For this review, take the finished solid that the model builds, in its own axes (mm). Round coordinates to 2 decimals unless told otherwise and drop trailing zeros. Write each loop counter-clockwise with the first axis right and the second up, starting at its lowest first coordinate (ties: lowest second). Pieces come first, ordered by that corner, then holes. Notation, with made-up numbers: (33.5, -38.75) -> (40.5, -38.75) arc R18 cw to (40.5, -15.75) -> close; hole circle Ø3 at (45.25, 81.5). An arc over 180 degrees is marked (long way). Answer in a Markdown table with one row per item. Add a question column.
```python
from build123d import *

# Parameters (mm, degrees)
SZKIC1_R                    = 1.5
SZKIC1_W                    = 45
SZKIC1_H                    = 5
SZKIC1_W_2                  = 5
SZKIC1_H_2                  = 55
DODANIE_WYCI_GNI_CIE3_DEPTH = 2


with BuildPart() as part:
    # Szkic1 → Dodanie-wyciągnięcie3 (new body)
    with BuildSketch(Plane.XY):
        with BuildLine():
            Line((-139.727293062, -79.5), (-120.189002398, -79.5))
            ThreePointArc((-120.189002398, -79.5), (-117.912369122, -78.544329486), (-117, -76.25))
            Line((-117, -76.25), (-117, -54.98069498))
            ThreePointArc((-117, -54.98069498), (-116.639537786, -54.110462214), (-115.76930502, -53.75))
            Line((-115.76930502, -53.75), (-102.427025017, -53.75))
            Line((-102.427025017, -53.75), (-87.218924948, -53.75))
            Line((-87.218924948, -53.75), (-36.25, -53.75))
            ThreePointArc((-36.25, -53.75), (-35.366116524, -54.116116524), (-35, -55))
            Line((-35, -55), (-35, -77.5))
            ThreePointArc((-35, -77.5), (0, -2.5), (-35, 72.5))
            Line((-35, 72.5), (-35, 51.25))
            ThreePointArc((-35, 51.25), (-35.366116524, 50.366116524), (-36.25, 50))
            Line((-36.25, 50), (-90.072974983, 50))
            Line((-90.072974983, 50), (-102.072974983, 50))
            Line((-102.072974983, 50), (-115.75, 50))
            ThreePointArc((-115.75, 50), (-116.633883476, 50.366116524), (-117, 51.25))
            Line((-117, 51.25), (-117, 73.75))
            ThreePointArc((-117, 73.75), (-117.366116524, 74.633883476), (-118.25, 75))
            Line((-118.25, 75), (-141.75, 75))
            ThreePointArc((-141.75, 75), (-142.633883476, 74.633883476), (-143, 73.75))
            Line((-143, 73.75), (-143, 51.25))
            ThreePointArc((-143, 51.25), (-143.366116524, 50.366116524), (-144.25, 50))
            Line((-144.25, 50), (-157.927025017, 50))
            Line((-157.927025017, 50), (-169.927025017, 50))
            Line((-169.927025017, 50), (-223.75, 50))
            ThreePointArc((-223.75, 50), (-224.633883476, 50.366116524), (-225, 51.25))
            Line((-225, 51.25), (-225, 72.5))
            ThreePointArc((-225, 72.5), (-260, -2.5), (-225, -77.5))
            Line((-225, -77.5), (-225, -55))
            ThreePointArc((-225, -55), (-224.633883476, -54.116116524), (-223.75, -53.75))
            Line((-223.75, -53.75), (-172.781075052, -53.75))
            Line((-172.781075052, -53.75), (-157.572974983, -53.75))
            Line((-157.572974983, -53.75), (-144.25, -53.75))
            ThreePointArc((-144.25, -53.75), (-143.366116524, -54.116116524), (-143, -55))
            Line((-143, -55), (-143, -76.237644119))
            ThreePointArc((-143, -76.237644119), (-142.040816528, -78.548140635), (-139.727293062, -79.5))
        make_face()
        with Locations((-229.818345238, 50.110219647)):
            Circle(SZKIC1_R, mode=Mode.SUBTRACT)
        with Locations((-229.818345238, -49.889780353)):
            Circle(SZKIC1_R, mode=Mode.SUBTRACT)
        with Locations(Location((-30.181654762, -49.889780353, 0), (0, 0, 180))):
            Circle(SZKIC1_R, mode=Mode.SUBTRACT)
        with Locations(Location((-30.181654762, 50.110219647, 0), (0, 0, 180))):
            Circle(SZKIC1_R, mode=Mode.SUBTRACT)
        with Locations((-187.5, 25)):
            Rectangle(SZKIC1_W, SZKIC1_H, mode=Mode.SUBTRACT)
        with Locations((-187.5, -25)):
            Rectangle(SZKIC1_W, SZKIC1_H, mode=Mode.SUBTRACT)
        with Locations((-72.5, -25)):
            Rectangle(SZKIC1_W, SZKIC1_H, mode=Mode.SUBTRACT)
        with Locations((-72.5, 25)):
            Rectangle(SZKIC1_W, SZKIC1_H, mode=Mode.SUBTRACT)
        with Locations((-15, 0)):
            Rectangle(SZKIC1_W_2, SZKIC1_H_2, mode=Mode.SUBTRACT)
        with Locations((-245, 0)):
            Rectangle(SZKIC1_W_2, SZKIC1_H_2, mode=Mode.SUBTRACT)
        with BuildLine():
            Line((-142.75, 20), (-117.25, 20))
            ThreePointArc((-117.25, 20), (-115.659009742, 19.340990258), (-115, 17.75))
            Line((-115, 17.75), (-115, -17.572974983))
            ThreePointArc((-115, -17.572974983), (-115.71085917, -19.28914083), (-117.427025017, -20))
            Line((-117.427025017, -20), (-142.75, -20))
            ThreePointArc((-142.75, -20), (-144.340990258, -19.340990258), (-145, -17.75))
            Line((-145, -17.75), (-145, 17.75))
            ThreePointArc((-145, 17.75), (-144.340990258, 19.340990258), (-142.75, 20))
        make_face(mode=Mode.SUBTRACT)
    extrude(amount=DODANIE_WYCI_GNI_CIE3_DEPTH)


solid = part.part
```
1. We need section D-D (y = -31). Write out the cut boundary in (x, z).
2. We need section C-C (x = -40). Write out the cut boundary in (y, z), plus the area to 4 significant figures.
3. For L1, parallel to Y at x = -53, z = 0.65; L2, parallel to X at y = -1.5, z = 1.95; L3, parallel to X at y = -13, z = 1.2, list the stretches that pass through material, from the lowest coordinate up. Write a range as [from, to].
4. Clearance check with flat-ended pins moving along their axes: pin 1 Ø2 at (x, y) = (-203.5, 24.5) entering from -Z; pin 2 Ø0.6 at (x, z) = (-194.5, 1) entering from +Y; pin 3 Ø1 at (x, z) = (-182.5, 1) entering from -Y; pin 4 Ø0.6 at (y, z) = (-25, 0.5) entering from +X. State where each tip first meets the part, or that it passes through.
5. We need section B-B (y = -0.5). Write out the cut boundary in (x, z), plus the area to 3 significant figures.
6. We need section A-A (x = -169.5). Write out the cut boundary in (y, z).
Response:
| question | item | result |
|---|---|---|
| 1 | outline | (-255.76, 0) -> (-4.24, 0) -> (-4.24, 2) -> (-255.76, 2) -> close |
| 2 | outline | (-53.75, 0) -> (50, 0) -> (50, 2) -> (-53.75, 2) -> close |
| 2 | area | 207.5 mm2 |
| 3 | L1 | [-53.75, -27.5], [-22.5, 22.5], [27.5, 50] |
| 3 | L2 | [-259.99, -247.5], [-242.5, -145], [-115, -17.5], [-12.5, -0.01] |
| 3 | L3 | [-259.44, -247.5], [-242.5, -145], [-115, -17.5], [-12.5, -0.56] |
| 4 | pin 1 | through |
| 4 | pin 2 | y = 50 |
| 4 | pin 3 | y = -53.75 |
| 4 | pin 4 | x = -2.55 |
| 5 | outline | (-259.98, 0) -> (-247.5, 0) -> (-247.5, 2) -> (-259.98, 2) -> close; (-242.5, 0) -> (-145, 0) -> (-145, 2) -> (-242.5, 2) -> close; (-115, 0) -> (-17.5, 0) -> (-17.5, 2) -> (-115, 2) -> close; (-12.5, 0) -> (-0.02, 0) -> (-0.02, 2) -> (-12.5, 2) -> close |
| 5 | area | 440 mm2 |
| 6 | outline | (-53.75, 0) -> (-27.5, 0) -> (-27.5, 2) -> (-53.75, 2) -> close; (-22.5, 0) -> (22.5, 0) -> (22.5, 2) -> (-22.5, 2) -> close; (27.5, 0) -> (50, 0) -> (50, 2) -> (27.5, 2) -> close |
